Here's how the part is built. I have some questions about the finished solid (model axes, mm). A direction names the side the tool comes from. Coordinates: 2 decimals unless noted, no trailing zeros. Write each loop counter-clockwise with the first axis right and the second up, starting at its lowest first coordinate (ties: lowest second). Pieces come first, ordered by that corner, then holes. Notation, with made-up numbers: M 15,12.25 L 52,12.25 A27 ccw 52,37.25 Z; hole C 32,34.5 d1. An arc over 180 degrees is marked long. Write each question's results on one line, items separated by ' | '. Start each with the question number.
from build123d import *

# Parameters (mm, degrees)
F0_R     = 1.6
F1_DEPTH = 2
F3_DEPTH = 0.5


with BuildPart() as f1:
    # F0 (on Top) → F1 (new body)
    with BuildSketch(Plane.XY):
        with BuildLine():
            Line((-19.906532, -14.3), (19.906532, -14.3))
            ThreePointArc((19.906532, -14.3), (20.880553, -14.046792), (21.607945, -13.351282))
            ThreePointArc((21.607945, -13.351282), (25.4, 0), (21.607945, 13.351282))
            ThreePointArc((21.607945, 13.351282), (20.880553, 14.046792), (19.906532, 14.3))
            Line((19.906532, 14.3), (-19.906532, 14.3))
            ThreePointArc((-19.906532, 14.3), (-20.880553, 14.046792), (-21.607945, 13.351282))
            ThreePointArc((-21.607945, 13.351282), (-25.4, 0), (-21.607945, -13.351282))
            ThreePointArc((-21.607945, -13.351282), (-20.880553, -14.046792), (-19.906532, -14.3))
        make_face()
        with Locations((-22, 0)):
            Circle(F0_R, mode=Mode.SUBTRACT)
    extrude(amount=F1_DEPTH)

    # F2 (on face) → F3 (cut)
    with BuildSketch(Plane.XY.offset(2)):
        with BuildLine():
            ThreePointArc((19.906532, -13.3), (20.393542, -13.173396), (20.757238, -12.825641))
            ThreePointArc((20.757238, -12.825641), (24.4, 0), (20.757238, 12.825641))
            ThreePointArc((20.757238, 12.825641), (20.393542, 13.173396), (19.906532, 13.3))
            Line((19.906532, 13.3), (-19.906532, 13.3))
            ThreePointArc((-19.906532, 13.3), (-20.393542, 13.173396), (-20.757238, 12.825641))
            ThreePointArc((-20.757238, 12.825641), (-24.4, 0), (-20.757238, -12.825641))
            ThreePointArc((-20.757238, -12.825641), (-20.393542, -13.173396), (-19.906532, -13.3))
            Line((-19.906532, -13.3), (19.906532, -13.3))
        make_face()
        with BuildLine():
            ThreePointArc((20.331885, 12.562821), (23.9, 0), (20.331885, -12.562821))
            ThreePointArc((20.331885, -12.562821), (20.150037, -12.736698), (19.906532, -12.8))
            Line((19.906532, -12.8), (-19.906532, -12.8))
            ThreePointArc((-19.906532, -12.8), (-20.150037, -12.736698), (-20.331885, -12.562821))
            ThreePointArc((-20.331885, -12.562821), (-23.9, 0), (-20.331885, 12.562821))
            ThreePointArc((-20.331885, 12.562821), (-20.150037, 12.736698), (-19.906532, 12.8))
            Line((-19.906532, 12.8), (19.906532, 12.8))
            ThreePointArc((19.906532, 12.8), (20.150037, 12.736698), (20.331885, 12.562821))
        make_face(mode=Mode.SUBTRACT)
    extrude(amount=-F3_DEPTH, mode=Mode.SUBTRACT)


solid = f1.part
1) I want a section at C-C, the plane y = -11.25. Write out the boundary of the cut face in (x, z), then the cut area to 3 significant figures.
2) For faces 5 (the cylindrical face through (-24.4, 0.2, 1.8)), 6 (the cylindrical face through (-20.868, 14.054, 0.986)), which set-ups out of +Z, -Z, +X, -X, +Y, -Y let a thin tool reach every point of the face, with its end or its side?
3) I want a section at A-A, the plane y = 0. Write out the boundary of the cut face in (x, z).
4) I want a section at D-D, the plane y = 9.75. Write out the boundary of the cut face in (x, z).
5) Please list where these lines run through material, in increasing order: line 1 (Y direction, x = -8.5, z = 1.8); line 2 (X direction, y = 10, z = 1.65); line 3 (Y direction, x = -22, z = 1.4). Write a range as [from, to].
6) I want a section at B-B, the plane z = 0.4. Write out the boundary of the cut face in (x, y).
7) We'd pull the mould along Y, two halves only. Please class faces 1 (the flat face through (0, 14, 2)), 2 (the flat face through (0, 14.3, 1)), 3 (the cylindrical face through (-23.9, -0.2, 1.8)), 4 (the cylindrical face through (-20.89, -14.04, 0.99)): pulls with the +Y half, pulls with the -Y half, needs draft (parallel to the pull), parting line crosses it, or undercut.
Output:
1) outline: M -22.77,0 L 22.77,0 L 22.77,2 L 21.65,2 L 21.65,1.5 L 21.09,1.5 L 21.09,2 L -21.09,2 L -21.09,1.5 L -21.65,1.5 L -21.65,2 L -22.77,2 Z | area: 90.5 mm2
2) face 5: +Z | face 6: +Z, -Z, -X, +Y
3) outline: M -25.4,0 L -23.6,0 L -23.6,2 L -23.9,2 L -23.9,1.5 L -24.4,1.5 L -24.4,2 L -25.4,2 Z; M -20.4,0 L 25.4,0 L 25.4,2 L 24.4,2 L 24.4,1.5 L 23.9,1.5 L 23.9,2 L -20.4,2 Z
4) outline: M -23.45,0 L 23.45,0 L 23.45,2 L 22.37,2 L 22.37,1.5 L 21.82,1.5 L 21.82,2 L -21.82,2 L -21.82,1.5 L -22.37,1.5 L -22.37,2 L -23.45,2 Z
5) line 1: y = [-14.3, -13.3], [-12.8, 12.8], [13.3, 14.3] | line 2: x = [-23.35, -22.26], [-21.71, 21.71], [22.26, 23.35] | line 3: y = [-12.69, -1.6], [1.6, 12.69]
6) outline: M -21.61,-13.35 A2 ccw -19.91,-14.3 L 19.91,-14.3 A2 ccw 21.61,-13.35 A25.4 ccw 21.61,13.35 A2 ccw 19.91,14.3 L -19.91,14.3 A2 ccw -21.61,13.35 A25.4 ccw Z; hole C -22,0 d3.2
7) face 1: needs draft | face 2: pulls with the +Y half | face 3: undercut | face 4: pulls with the -Y half
